```python
from build123d import *

# Parameters (mm, degrees)
SKETCH_1_R             = 5
EXTRUDE_1_DEPTH        = 106
SKETCH_2_R             = 8
EXTRUDE_2_DEPTH        = 4
SKETCH_4_W             = 1.5
SKETCH_4_H             = 19.56005024
CUT_EXTRUDE_1_DEPTH    = 2
HOLE_WIZARD_M8_1_D     = 6.8
HOLE_WIZARD_M8_1_DEPTH = 15
HOLE_WIZARD_M8_1_TIP   = 2.042926105


with BuildPart() as part:
    # 草图1 → 凸台-拉伸1 (new body)
    with BuildSketch(Plane.XY):
        Circle(SKETCH_1_R)
    extrude(amount=EXTRUDE_1_DEPTH)

    # 草图2 → 凸台-拉伸2 (add)
    with BuildSketch(Plane.XY.offset(106)):
        Circle(SKETCH_2_R)
    extrude(amount=EXTRUDE_2_DEPTH)

    # 草图4 → 切除-拉伸1 (cut)
    with BuildSketch(Plane.XY.offset(110)):
        Rectangle(SKETCH_4_W, SKETCH_4_H)
    extrude(amount=-CUT_EXTRUDE_1_DEPTH, mode=Mode.SUBTRACT)

    # M8 螺纹孔的螺纹孔钻头1
    with Locations(Plane(origin=(0, 0, 0), x_dir=(-1, 0, 0), z_dir=(0, 0, -1))):
        with Locations((0, 0)):
            Hole(HOLE_WIZARD_M8_1_D / 2, depth=HOLE_WIZARD_M8_1_DEPTH)
            with Locations((0, 0, -(HOLE_WIZARD_M8_1_DEPTH + HOLE_WIZARD_M8_1_TIP / 2))):  # 118° drill point
                Cone(0, HOLE_WIZARD_M8_1_D / 2, HOLE_WIZARD_M8_1_TIP, mode=Mode.SUBTRACT)


solid = part.part
```
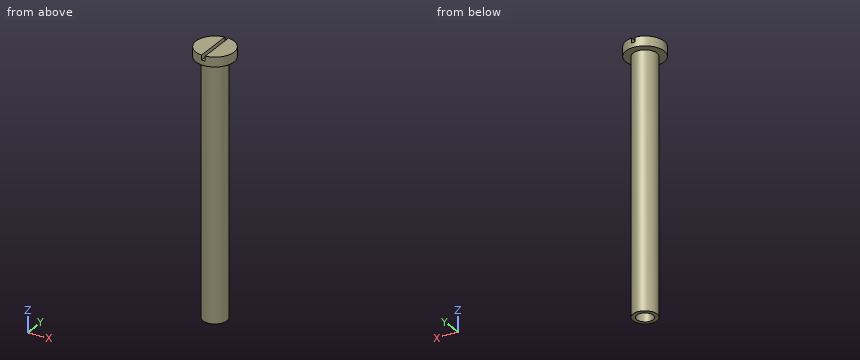
Can you work these out from the model? Positions are in its coordinate system, mm. Round coordinates to 2 decimals unless told otherwise and drop trailing zeros. Loops run counter-clockwise (first coordinate to the right, second up) from the corner with the lowest first, then second, coordinate; pieces in that order, holes last.
Item 1: Will these pins go through, and if not, where does the flat tip stop? pin 1 Ø5 at (x, y) = (4, 6) entering from -Z; pin 2 Ø1.5 at (y, z) = (4.5, 50.5) entering from +X; pin 3 Ø1 at (y, z) = (-3.5, 109) entering from +X; pin 4 Ø1.5 at (x, y) = (-2, 1.5) entering from -Z.
Item 2: Please list where these lines run through material, in increasing order: L1, parallel to Y at x = 0, z = 7; L2, parallel to Z at x = -2.5, y = -5.25; L3, parallel to X at y = 1.75, z = 103.
Item 3: Suppose I cut it at C-C, the plane z = 66. Write out the boundary of the cut face in (x, y), then the cut area to 3 significant figures.
Item 4: Suppose I cut it at B-B, the plane y = 6. Write out the boundary of the cut face in (x, z).
Item 5: Suppose I cut it at A-A, the plane z = 14. Write out the boundary of the cut face in (x, y), then the cut area to 3 significant figures.
Reported:
1. pin 1: stops at z = 0
1. pin 2: stops at x = 3.31
1. pin 3: stops at x = 7.42
1. pin 4: stops at z = 15.09
2. L1: y = -5 to -3.4, 3.4 to 5
2. L2: z = 106 to 110
2. L3: x = -4.68 to 4.68
3. outline: circle Ø10 at (0, 0)
3. area: 78.5 mm2
4. outline: (-5.29, 106) - (5.29, 106) - (5.29, 110) - (0.75, 110) - (0.75, 108) - (-0.75, 108) - (-0.75, 110) - (-5.29, 110) - close
5. outline: circle Ø10 at (0, 0); hole circle Ø6.8 at (0, 0)
5. area: 42.2 mm2
